Input: part model. Units: mm. Frame: model coordinates. Round coordinates to 2 decimals unless told otherwise and drop trailing zeros. Loops run counter-clockwise (first coordinate to the right, second up) from the corner with the lowest first, then second, coordinate; pieces in that order, holes last. Notation, with made-up numbers: M -11,6 L 36,6 A26 cw 36,44 Z; hole C -21.75,53.5 d2. An arc over 180 degrees is marked long. Return JSON: item names as keys, results as strings. Group by question number.
1) Section B-B (x = 0). Output: boundary loops of the cut face in (y, z).
2) Section A-A (z = 3). Output: boundary loops of the cut face in (x, y).
3) Mould query, pull axis Y, two halves, no side actions, for faces 1 (the face through (76.95, 59.37, 14.03)), 2 (the face through (81, -34, 12.15)), 3 (the face through (-19.9, 89.617, 6.828)), 4 (the face through (77.36, -59.85, 6.61)). Classes: +Y half, -Y half, draft (parallel to the pull), parting line (faces both ways), or undercut.
4) Contact query for flat-ended pins moving along their axis: P1, Ø10, axis at x = 64.5, y = -27.5, coming from the -Z side; P2, Ø6, axis at x = 22.5, z = 5, coming from the -Y side; P3, Ø4, axis at y = 44.5, z = 10, coming from the -X side. Output: stop coordinate, or through.
5) Material intervals for line 1 (Y direction, x = 0, z = 10); line 2 (Y direction, x = 0, z = 7.25); line 3 (X direction, y = -1, z = 12), sorted ascending. Write a range as from..to.
Autodesk Inventor part; units mm, degrees
ref_plane "Work Plane1" through (0, 0, 8.9) normal (0, 0, 1) x (1, 0, 0)
ref_plane "YZ Plane" through (0, 0, 0) normal (1, 0, 0) x (0, 1, 0)
ref_plane "XZ Plane" through (0, 0, 0) normal (0, 1, 0) x (-1, 0, 0)
sketch "Sketch1" plane through (0, 0, 0) normal (0, 0, 1) x (1, 0, 0)
  line L0 (95.8, -44.0209) -> (95.8, 44.0209)
  line L1 (95.8, 44.0209) -> (0, 126.2524)
  circle A0 centre (0, 0) radius 91.8
  line L2 (-95.8, 44.0209) -> (-95.8, -44.0209)
  line L3 (0, -126.2524) -> (95.8, -44.0209)
  line L4 (0, 126.2524) -> (-95.8, 44.0209)
  line L5 (-95.8, -44.0209) -> (0, -126.2524)
  dimension "d47" = 183.6
extrude "Extrusion3" add sketch "Sketch1" along normal blind 14.65
ref_plane "Work Plane1" through (0, 0, 8.9) normal (0, 0, 1) x (1, 0, 0)
sketch "Sketch2" plane through (0, 0, 8.9) normal (0, 0, 1) x (1, 0, 0)
  circle A0 centre (0, 0) radius 91.8
  circle A1 centre (0, 0) radius 87.5
  circle A2 centre (0, 0) radius 91.8
  line L0 (95.8, -44.0209) -> (95.8, 44.0209)
  line L1 (0, -126.2524) -> (95.8, -44.0209)
  line L2 (-95.8, -44.0209) -> (0, -126.2524)
  line L3 (-95.8, 44.0209) -> (-95.8, -44.0209)
  line L4 (0, 126.2524) -> (-95.8, 44.0209)
  line L5 (95.8, 44.0209) -> (0, 126.2524)
  dimension "d54" = 4.3
extrude "Extrusion2" add sketch "Sketch2" along normal blind 5.75 contours A1
sketch "Sketch3" plane through (0, 0, 14.65) normal (0, 0, 1) x (1, 0, 0)
  line L0 (-79.5276, -36.4912) -> (-83.4629, -38.2253)
  circle A0 centre (0, 0) radius 89
  circle A1 centre (0, 0) radius 89
  circle A2 centre (0, 0) radius 91.8
  circle A3 centre (0, 0) radius 91.8
  line L1 (95.8, -44.0209) -> (0, -126.2524)
  line L2 (0, -126.2524) -> (-95.8, -44.0209)
  line L3 (-95.8, -44.0209) -> (-95.8, 44.0209)
  line L4 (-95.8, 44.0209) -> (0, 126.2524)
  line L5 (0, 126.2524) -> (95.8, 44.0209)
  line L6 (95.8, 44.0209) -> (95.8, -44.0209)
  circle A4 centre (0, 0) radius 91.8
  line L7 (95.8, -44.0209) -> (95.8, 44.0209)
  line L8 (0, -126.2524) -> (95.8, -44.0209)
  line L9 (-95.8, -44.0209) -> (0, -126.2524)
  line L10 (-95.8, 44.0209) -> (-95.8, -44.0209)
  line L11 (0, 126.2524) -> (-95.8, 44.0209)
  line L12 (95.8, 44.0209) -> (0, 126.2524)
  circle A5 centre (0, 0) radius 87.5
  circle A6 centre (0, 0) radius 87.5
  line L13 (-84.6557, -35.5056) -> (-80.6929, -33.8366)
  point P0 (-84.0051, -35.376)
  point P1 (-83.4629, -38.2253)
  point P2 (-81.2652, -37.2569)
  point P3 (-84.6557, -35.5056)
  point P4 (-83.4629, -38.2253)
  dimension "d55" = 2.93
extrude "Extrusion1" add sketch "Sketch3" against normal blind 2.5 contours A5 L13 A0 L0 | A0 L13 A2 L0 picked at (12.3499, -86.9619) picked at (90.2127, 8.8539)
fillet "Fillet9" radius 0.8 1 edges at (-82.6743, -34.6711, 12.15)
fillet "Fillet8" radius 0.8 1 edges at (-81.4953, -37.3583, 12.15)
fillet "Fillet7" radius 0.8 2 edges at (-81.4953, -37.3583, 14.65) (-84.0703, -36.8703, 14.65)
fillet "Fillet7" radius 0.8 2 edges at (-80.1212, -35.1687, 14.65) (-82.6743, -34.6711, 14.65)
fillet "Fillet6" radius 8.7504 1 edges at (-95.8, 44.0209, 7.325)
fillet "Fillet5" radius 8.7504 1 edges at (-95.8, -44.0209, 7.325)
fillet "Fillet4" radius 8.7504 1 edges at (95.8, 44.0209, 7.325)
fillet "Fillet3" radius 8.7504 1 edges at (95.8, -44.0209, 7.325)
fillet "Fillet2" radius 95.8 1 edges at (0, -126.2524, 7.325)
fillet "Fillet1" radius 95.8 1 edges at (0, 126.2524, 7.325)
chamfer "Chamfer1" distance 1.25 angle 45 12 edges at (0, -95.8, 14.65) (-95.0007, 43.6536, 14.65) (77.573, -59.6663, 14.65) (-77.573, 59.6663, 14.65) (95.0007, -43.6536, 14.65) (0, 95.8, 14.65) (77.573, 59.6663, 14.65) (-95.0007, -43.6536, 14.65) (95.0007, 43.6536, 14.65) (-95.8, 0, 14.65) (-77.573, -59.6663, 14.65) (95.8, 0, 14.65)
hole "Hole4" at (-89.8894, 41.3049, 14.65) direction (0, 0, -1) diameter 4 depth 14.65
hole "Hole3" at (89.8894, -41.3049, 14.65) direction (0, 0, -1) diameter 4 depth 14.65
sketch "Sketch5" plane through (0, 0, 14.65) normal (0, 0, 1) x (1, 0, 0)
  point P0 (89.8894, -41.3049)
hole "Hole2" at (-89.8894, -41.3049, 14.65) direction (0, 0, -1) diameter 4 depth 14.65
sketch "Sketch4" plane through (0, 0, 14.65) normal (0, 0, 1) x (1, 0, 0)
  point P0 (-89.8894, 41.3049)
hole "Hole1" at (89.8894, 41.3049, 14.65) direction (0, 0, -1) diameter 4 depth 14.65
sketch "Sketch8" plane through (0, 0, 0) normal (1, 0, 0) x (0, 1, 0)
  line L0 (-91, 1) -> (-93.3, 1)
  line L1 (-88, 1.25) -> (-90, 1.25)
  line L2 (-93.3, 1) -> (-93.3, 0)
  line L3 (-90, 4.25) -> (-91, 4.25)
  line L4 (-90, 4.25) -> (-90, 1.25)
  line L5 (-88, 0) -> (-93.3, 0)
  line L6 (-91, 4.25) -> (-91, 1)
  line L7 (-88, 1.25) -> (-88, 0)
  line L8 (0, 0) -> (0, -10)
revolve "Revolution1" [suppressed]
sketch "Sketch9" plane through (0, 0, 0) normal (1, 0, 0) x (0, 1, 0)
  line L0 (-91, 1) -> (-93.3, 1)
  line L1 (-93.3, 1) -> (-93.3, 0)
  line L2 (0, 0) -> (-93.3, 0)
  line L3 (-91, 4.25) -> (-91, 1)
  line L4 (0, 4.25) -> (-91, 4.25)
  line L5 (0, 0) -> (0, 4.25)
  line L6 (0, 0) -> (0, -10)
revolve "Revolution2" [suppressed]
sketch "Sketch10" plane through (0, 0, 0) normal (1, 0, 0) x (0, 1, 0)
  line L0 (0, 4.25) -> (90, 4.25)
  line L1 (90, 4.25) -> (90, 1.25)
  line L2 (90, 1.25) -> (88, 1.25)
  line L3 (88, 1.25) -> (88, 0)
  line L4 (88, 0) -> (0, 0)
  line L5 (0, 0) -> (0, 4.25)
  line L6 (0, 4.25) -> (0, 0)
revolve "Revolution3" [suppressed]
sketch "Sketch6" plane through (0, 0, 14.65) normal (0, 0, 1) x (1, 0, 0)
  point P0 (-89.8894, -41.3049)
sketch "Sketch7" plane through (0, 0, 14.65) normal (0, 0, 1) x (1, 0, 0)
  point P0 (89.8894, 41.3049)
properties part number "Body_3DPrint"
Returned:
{
 "1": {"outline": "M -95.8,0 L -91.8,0 L -91.8,12.15 L -87.5,12.15 L -87.5,8.9 L 87.5,8.9 L 87.5,12.15 L 91.8,12.15 L 91.8,0 L 95.8,0 L 95.8,13.4 L 94.55,14.65 L -94.55,14.65 L -95.8,13.4 Z"},
 "2": {"outline": "M -95.8,-40 A8.75 ccw -92.75,-46.64 L -62.4,-72.69 A95.8 ccw 62.4,-72.69 L 92.75,-46.64 A8.75 ccw 95.8,-40 L 95.8,40 A8.75 ccw 92.75,46.64 L 62.4,72.69 A95.8 ccw -62.4,72.69 L -92.75,46.64 A8.75 ccw -95.8,40 Z; hole C -89.89,-41.3 d4; hole C -89.89,41.3 d4; hole C 0,0 d183.6; hole C 89.89,-41.3 d4; hole C 89.89,41.3 d4"},
 "3": {"face 1": "+Y half", "face 2": "undercut", "face 3": "undercut", "face 4": "-Y half"},
 "4": {"P1": "stops at z = 8.9", "P2": "stops at y = -93.79", "P3": "stops at x = -95.44"},
 "5": {"line 1": "y = -95.8..-91.8, -87.5..87.5, 91.8..95.8", "line 2": "y = -95.8..-91.8, 91.8..95.8", "line 3": "x = -95.8..-91.79, -87.49..87.49, 91.79..95.8"}
}
